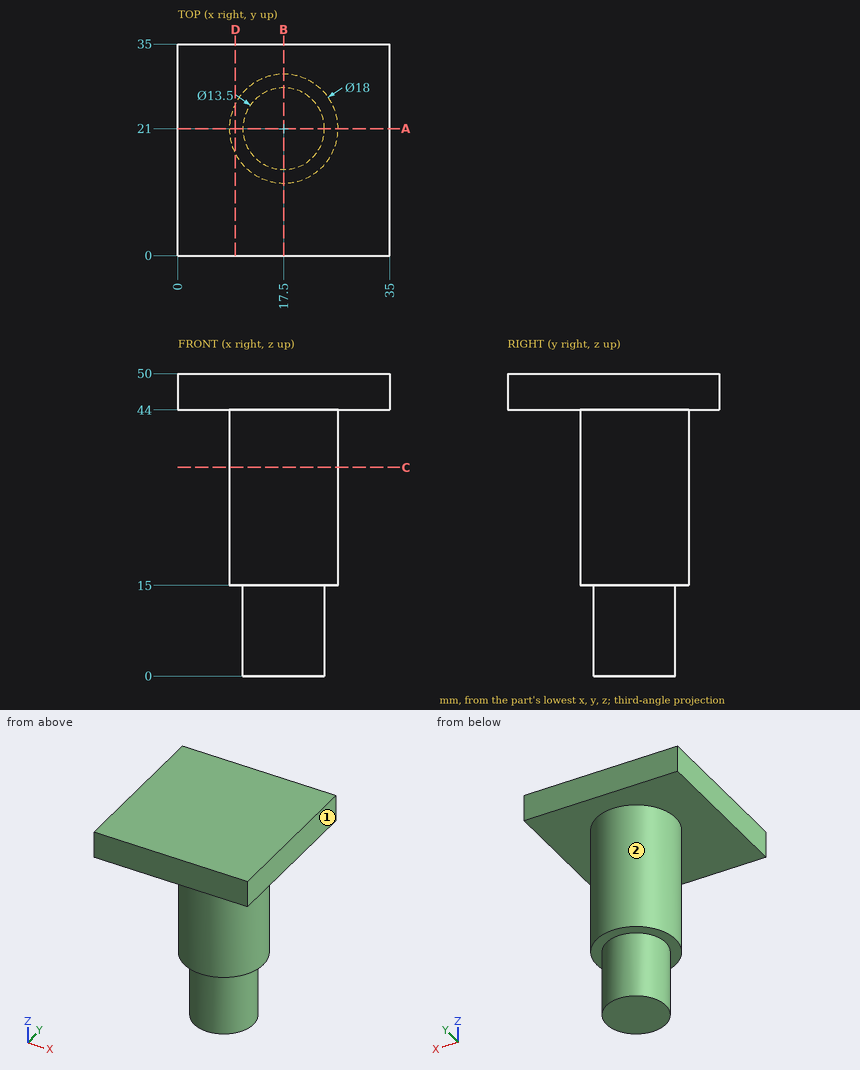
Geometry: see drawing. Coordinates: mm, zero at the bounding-box minimum. A direction names the side the tool comes from. Give positions to 0.01 mm unless a question says otherwise; leave off trailing zeros. Loops run counter-clockwise (first coordinate to the right, second up) from the corner with the lowest first, then second, coordinate; pieces in that order, holes last. Notation, with made-up numbers: (24.25, 34) -> (67.25, 34) arc R15 ccw to (67.25, 42) -> close; hole circle Ø7 at (66, 42.25). An arc over 180 degrees is marked (long way). Answer as a JSON object with one key per item and string values. Group by question number.
Item 1: Line query: probe 1 along Z at (x, y) = (8.5, 25); probe 2 along Z at (x, y) = (25, 22.5); probe 3 along X at (y, z) = (29, 25.5). Output: solid intervals per line, ascending.
Item 2: Cut plane B-B, the plane x = 17.5. Return the cut outline in (y, z).
Item 3: Reachability of the marked faces 1 and 2 from +Z, -Z, +X, -X, +Y, -Y: full face, straight path, thin tool, end or side. Return the list, or none.
Item 4: Pin query (flat end, axial travel): P1, Ø3, axis at y = 19, z = 29.5, coming from the +X side; P2, Ø5, axis at y = 29, z = 17.5, coming from the +X side; P3, Ø12, axis at x = 11, z = 16, coming from the +Y side. Return the tip coordinate at first contact, or that it passes through.
Item 5: Cut plane D-D, the plane x = 9.5. Return the cut outline in (y, z), and give its area (3 significant figures).
Item 6: Cut plane C-C, the plane z = 34.5. Return the cut outline in (x, y), and give its area (3 significant figures).
Item 7: Cut plane A-A, the plane y = 21. Return the cut outline in (x, z), and give its area (4 significant figures).
Checks:
{
 "1": {"probe 1": "z = 44 to 50", "probe 2": "z = 15 to 50", "probe 3": "x = 13.38 to 21.62"},
 "2": {"outline": "(0, 44) -> (12, 44) -> (12, 15) -> (14.25, 15) -> (14.25, 0) -> (27.75, 0) -> (27.75, 15) -> (30, 15) -> (30, 44) -> (35, 44) -> (35, 50) -> (0, 50) -> close"},
 "3": {"face 1": "+Z, -Z, +X, +Y, -Y", "face 2": "-Z"},
 "4": {"P1": "stops at x = 26.49", "P2": "stops at x = 24.62", "P3": "stops at y = 29.99"},
 "5": {"outline": "(0, 44) -> (16.88, 44) -> (16.88, 15) -> (25.12, 15) -> (25.12, 44) -> (35, 44) -> (35, 50) -> (0, 50) -> close", "area": "449 mm²"},
 "6": {"outline": "circle Ø18 at (17.5, 21)", "area": "254 mm²"},
 "7": {"outline": "(0, 44) -> (8.5, 44) -> (8.5, 15) -> (10.75, 15) -> (10.75, 0) -> (24.25, 0) -> (24.25, 15) -> (26.5, 15) -> (26.5, 44) -> (35, 44) -> (35, 50) -> (0, 50) -> close", "area": "934.5 mm²"}
}
